from build123d import *

# Parameters (mm, degrees)
F0_R     = 5
F1_DEPTH = 5
F3_DEPTH = 10


with BuildPart() as f1:
    # F0 (on Front) → F1 (new body, symmetric)
    with BuildSketch(Plane.XZ):
        with BuildLine():
            Line((-8.519582, 16.38709), (-7.378114, 13.63134))
            ThreePointArc((-7.378114, 13.63134), (-8.611339, 12.887779), (-9.770235, 12.032976))
            Line((-9.770235, 12.032976), (-11.879394, 14.142136))
            ThreePointArc((-11.879394, 14.142136), (-14.142136, 14.142136), (-14.142136, 11.879394))
            Line((-14.142136, 11.879394), (-12.032976, 9.770235))
            ThreePointArc((-12.032976, 9.770235), (-12.887779, 8.611339), (-13.63134, 7.378114))
            Line((-13.63134, 7.378114), (-16.38709, 8.519582))
            ThreePointArc((-16.38709, 8.519582), (-18.477591, 7.653669), (-17.611677, 5.563168))
            Line((-17.611677, 5.563168), (-14.855927, 4.421699))
            ThreePointArc((-14.855927, 4.421699), (-15.202172, 3.0239), (-15.417198, 1.6))
            Line((-15.417198, 1.6), (-18.4, 1.6))
            ThreePointArc((-18.4, 1.6), (-20, 0), (-18.4, -1.6))
            Line((-18.4, -1.6), (-15.417198, -1.6))
            ThreePointArc((-15.417198, -1.6), (-15.202172, -3.0239), (-14.855927, -4.421699))
            Line((-14.855927, -4.421699), (-17.611677, -5.563168))
            ThreePointArc((-17.611677, -5.563168), (-18.477591, -7.653669), (-16.38709, -8.519582))
            Line((-16.38709, -8.519582), (-13.63134, -7.378114))
            ThreePointArc((-13.63134, -7.378114), (-12.887779, -8.611339), (-12.032976, -9.770235))
            Line((-12.032976, -9.770235), (-14.142136, -11.879394))
            ThreePointArc((-14.142136, -11.879394), (-14.142136, -14.142136), (-11.879394, -14.142136))
            Line((-11.879394, -14.142136), (-9.770235, -12.032976))
            ThreePointArc((-9.770235, -12.032976), (-8.611339, -12.887779), (-7.378114, -13.63134))
            Line((-7.378114, -13.63134), (-8.519582, -16.38709))
            ThreePointArc((-8.519582, -16.38709), (-7.653669, -18.477591), (-5.563168, -17.611677))
            Line((-5.563168, -17.611677), (-4.421699, -14.855927))
            ThreePointArc((-4.421699, -14.855927), (-3.0239, -15.202172), (-1.6, -15.417198))
            Line((-1.6, -15.417198), (-1.6, -18.4))
            ThreePointArc((-1.6, -18.4), (0, -20), (1.6, -18.4))
            Line((1.6, -18.4), (1.6, -15.417198))
            ThreePointArc((1.6, -15.417198), (3.0239, -15.202172), (4.421699, -14.855927))
            Line((4.421699, -14.855927), (5.563168, -17.611677))
            ThreePointArc((5.563168, -17.611677), (7.653669, -18.477591), (8.519582, -16.38709))
            Line((8.519582, -16.38709), (7.378114, -13.63134))
            ThreePointArc((7.378114, -13.63134), (8.611339, -12.887779), (9.770235, -12.032976))
            Line((9.770235, -12.032976), (11.879394, -14.142136))
            ThreePointArc((11.879394, -14.142136), (14.142136, -14.142136), (14.142136, -11.879394))
            Line((14.142136, -11.879394), (12.032976, -9.770235))
            ThreePointArc((12.032976, -9.770235), (12.887779, -8.611339), (13.63134, -7.378114))
            Line((13.63134, -7.378114), (16.38709, -8.519582))
            ThreePointArc((16.38709, -8.519582), (18.477591, -7.653669), (17.611677, -5.563168))
            Line((17.611677, -5.563168), (14.855927, -4.421699))
            ThreePointArc((14.855927, -4.421699), (15.202172, -3.0239), (15.417198, -1.6))
            Line((15.417198, -1.6), (18.4, -1.6))
            ThreePointArc((18.4, -1.6), (20, 0), (18.4, 1.6))
            Line((18.4, 1.6), (15.417198, 1.6))
            ThreePointArc((15.417198, 1.6), (15.202172, 3.0239), (14.855927, 4.421699))
            Line((14.855927, 4.421699), (17.611677, 5.563168))
            ThreePointArc((17.611677, 5.563168), (18.477591, 7.653669), (16.38709, 8.519582))
            Line((16.38709, 8.519582), (13.63134, 7.378114))
            ThreePointArc((13.63134, 7.378114), (12.887779, 8.611339), (12.032976, 9.770235))
            ThreePointArc((12.032976, 9.770235), (10.960155, 10.960155), (9.770235, 12.032976))
            ThreePointArc((9.770235, 12.032976), (8.611339, 12.887779), (7.378114, 13.63134))
            Line((7.378114, 13.63134), (8.519582, 16.38709))
            ThreePointArc((8.519582, 16.38709), (7.653669, 18.477591), (5.563168, 17.611677))
            Line((5.563168, 17.611677), (4.421699, 14.855927))
            ThreePointArc((4.421699, 14.855927), (3.0239, 15.202172), (1.6, 15.417198))
            Line((1.6, 15.417198), (1.6, 18.4))
            ThreePointArc((1.6, 18.4), (0, 20), (-1.6, 18.4))
            Line((-1.6, 18.4), (-1.6, 15.417198))
            ThreePointArc((-1.6, 15.417198), (-3.0239, 15.202172), (-4.421699, 14.855927))
            Line((-4.421699, 14.855927), (-5.563168, 17.611677))
            ThreePointArc((-5.563168, 17.611677), (-7.653669, 18.477591), (-8.519582, 16.38709))
        make_face()
        Circle(F0_R, mode=Mode.SUBTRACT)
        with BuildLine():
            Line((11.879394, 14.142136), (9.770235, 12.032976))
            ThreePointArc((9.770235, 12.032976), (10.960155, 10.960155), (12.032976, 9.770235))
            Line((12.032976, 9.770235), (14.142136, 11.879394))
            ThreePointArc((14.142136, 11.879394), (14.142136, 14.142136), (11.879394, 14.142136))
        make_face()
    extrude(amount=F1_DEPTH, both=True)

    # F2 (on face) → F3 (cut)
    with BuildSketch(Plane.XZ.offset(5)):
        with BuildLine():
            ThreePointArc((-6.190476, 11.431448), (-9.192388, 9.192388), (-11.431448, 6.190476))
            ThreePointArc((-11.431448, 6.190476), (-11.656508, 5.614049), (-11.733093, 5))
            Line((-11.733093, 5), (-4.153312, 5))
            ThreePointArc((-4.153312, 5), (-3.887479, 5.209367), (-3.611111, 5.404616))
            ThreePointArc((-3.611111, 5.404616), (-2.795207, 6.304803), (-2.5, 7.483315))
            Line((-2.5, 7.483315), (-2.5, 9.233093))
            ThreePointArc((-2.5, 9.233093), (-3.720584, 11.380904), (-6.190476, 11.431448))
        make_face()
        with BuildLine():
            Line((-4.153312, 5), (-11.733093, 5))
            ThreePointArc((-11.733093, 5), (-11.00086, 3.232233), (-9.233093, 2.5))
            Line((-9.233093, 2.5), (-7.483315, 2.5))
            ThreePointArc((-7.483315, 2.5), (-6.304803, 2.795207), (-5.404616, 3.611111))
            ThreePointArc((-5.404616, 3.611111), (-4.829156, 4.350776), (-4.153312, 5))
        make_face()
        with BuildLine():
            ThreePointArc((6.190476, 11.431448), (3.720584, 11.380904), (2.5, 9.233093))
            Line((2.5, 9.233093), (2.5, 7.483315))
            ThreePointArc((2.5, 7.483315), (2.795207, 6.304803), (3.611111, 5.404616))
            ThreePointArc((3.611111, 5.404616), (4.596194, 4.596194), (5.404616, 3.611111))
            ThreePointArc((5.404616, 3.611111), (6.304803, 2.795207), (7.483315, 2.5))
            Line((7.483315, 2.5), (9.233093, 2.5))
            ThreePointArc((9.233093, 2.5), (11.380904, 3.720584), (11.431448, 6.190476))
            ThreePointArc((11.431448, 6.190476), (9.192388, 9.192388), (6.190476, 11.431448))
        make_face()
        with BuildLine():
            Line((-7.483315, -2.5), (-9.233093, -2.5))
            ThreePointArc((-9.233093, -2.5), (-11.380904, -3.720584), (-11.431448, -6.190476))
            ThreePointArc((-11.431448, -6.190476), (-9.192388, -9.192388), (-6.190476, -11.431448))
            ThreePointArc((-6.190476, -11.431448), (-3.720584, -11.380904), (-2.5, -9.233093))
            Line((-2.5, -9.233093), (-2.5, -7.483315))
            ThreePointArc((-2.5, -7.483315), (-2.795207, -6.304803), (-3.611111, -5.404616))
            ThreePointArc((-3.611111, -5.404616), (-4.596194, -4.596194), (-5.404616, -3.611111))
            ThreePointArc((-5.404616, -3.611111), (-6.304803, -2.795207), (-7.483315, -2.5))
        make_face()
        with BuildLine():
            ThreePointArc((5.404616, -3.611111), (4.596194, -4.596194), (3.611111, -5.404616))
            ThreePointArc((3.611111, -5.404616), (2.795207, -6.304803), (2.5, -7.483315))
            Line((2.5, -7.483315), (2.5, -9.233093))
            ThreePointArc((2.5, -9.233093), (3.720584, -11.380904), (6.190476, -11.431448))
            ThreePointArc((6.190476, -11.431448), (9.192388, -9.192388), (11.431448, -6.190476))
            ThreePointArc((11.431448, -6.190476), (11.380904, -3.720584), (9.233093, -2.5))
            Line((9.233093, -2.5), (7.483315, -2.5))
            ThreePointArc((7.483315, -2.5), (6.304803, -2.795207), (5.404616, -3.611111))
        make_face()
    extrude(amount=-F3_DEPTH, mode=Mode.SUBTRACT)


solid = f1.part
Model file for the job. Use its own axes, mm. A direction names the side the tool comes from. Give positions to 0.01 mm unless a question says otherwise; leave off trailing zeros. Write each loop counter-clockwise with the first axis right and the second up, starting at its lowest first coordinate (ties: lowest second). Pieces come first, ordered by that corner, then holes. Notation, with made-up numbers: M -15.75,26 L 35.25,26 A29 cw 35.25,57 Z; hole C 54,-26 d3. An arc over 180 degrees is marked long. One line per item, written item: value. Start each with the question number.
Q1. Saw through at A-A, the plane z = 0. Write the cut outline in (x, y).
Q2. Two-plate mould, pull along X, no slides. Class faces 1 (the flat face through (-17, 0, -1.6)), 2 (the cylindrical face through (-2.8, -0.1, 6.3)), 3 (the cylindrical face through (-20, 0, 0)): +X half, -X half, draft (parallel to the pull), parting line (faces both ways), or undercut.
Q3. Saw through at C-C, the plane x = -13. Write the cut outline in (y, z), plus the area to 3 significant figures.
Q4. Drop flat-ended pins along their axis: pin 1 Ø0.9 at (y, z) = (0.5, -8.5) entering from +X; pin 2 Ø0.9 at (y, z) = (-0.5, 16.5) entering from +X; pin 3 Ø1.9 at (x, y) = (8, 1.5) entering from -Z. Give the stop position or say it passes through.
Q5. Saw through at B-B, the plane z = -17. Write the cut outline in (x, y), plus the area to 3 significant figures.
Q6. 3-axis set-ups, long thin cutter, end or side, ignore diameter. For faces 4 (the flat face through (-16.215, -0.07, -4.984)), 5 (the cylindrical face through (6.3, -0.1, 2.8)), 6 (the flat face through (-1.6, 0, 17)), 7 (the flat face through (-10.84, -0.07, -13.1)): which of +Z, -Z, +X, -X, +Y, -Y reach the whole face in a straight line?
Q7. Probe probe 1 along Z at (x, y) = (0, 1.25); probe 2 along Z at (x, y) = (-4.5, -2.5); probe 3 along Z at (x, y) = (12.5, 0.75). List the from-to ranges inside material, lowest first. Write a range as [from, to].
Q8. Saw through at D-D, the plane y = 3. State how many separate pieces and enclosed holes the cut face has, plus the area to 3 significant figures.
Output values:
1. outline: M -20,-5 L -5,-5 L -5,5 L -20,5 Z; M 5,-5 L 20,-5 L 20,5 L 5,5 Z
2. face 1: draft
2. face 2: undercut
2. face 3: -X half
3. outline: M -5,-14.61 L 5,-14.61 L 5,-10.74 L -5,-10.74 Z; M -5,-8.44 L 5,-8.44 L 5,8.44 L -5,8.44 Z; M -5,10.74 L 5,10.74 L 5,14.61 L -5,14.61 Z
3. area: 246 mm²
4. pin 1: stops at x = 18.24
4. pin 2: stops at x = 8.64
4. pin 3: stops at z = -18.6
5. outline: M -8.64,-5 L -5.31,-5 L -5.31,5 L -8.64,5 Z; M -1.6,-5 L 1.6,-5 L 1.6,5 L -1.6,5 Z; M 5.31,-5 L 8.64,-5 L 8.64,5 L 5.31,5 Z
5. area: 98.6 mm²
6. face 4: -X, +Y, -Y
6. face 5: +Y, -Y
6. face 6: +Z, +Y, -Y
6. face 7: -Z, +Y, -Y
7. probe 1: z = [-20, -5], [5, 20]
7. probe 2: z = [-15.04, -11.68], [-4.69, -2.18], [2.18, 4.69], [11.68, 15.04]
7. probe 3: z = [-14.53, -10.24], [-9.17, 9.17], [10.24, 14.53]
8. separate pieces: 1
8. enclosed holes: 5
8. area: 652 mm²
